Here's how the part is built. I have some questions about the finished solid (model axes, mm). A direction names the side the tool comes from. Coordinates: 2 decimals unless noted, no trailing zeros. Order: outer loops, then holes, each group sorted by start corner. A loop starts at its lowest first (then second) coordinate and runs counter-clockwise, first axis right, second up. Notation, with made-up numbers: (40.5, -21) - (60.5, -21) arc R35 cw to (60.5, 12) - close; hole circle Ø5 at (16.25, 25.5). An arc over 180 degrees is marked (long way). Answer as CSV lines item,"result". Start each with the question number.
Item 1: Imagine slicing it at A-A on y = 5. List the corners of the cut face in (x, z) for me, and give its area (3 significant figures).
Item 2: On a 3-axis mill with a long thin cutter (end or side, diameter ignored), from which of +Z, -Z, +X, -X, +Y, -Y can I reach the whole of each face in a straight line? I mean faces 1 (the face through (29.007, 27.888, 5.378)), 2 (the face through (-19.2, 27.9, 22.4)), 3 (the face through (-28, 0, 2)), 4 (the face through (25.659, 3.944, -14.557)), 5 (the face through (25.44, 3.94, 14.94)). Say none if no direction works.
Item 3: We'd pull the mould along X, two halves only. Please class faces 6 (the face through (-14, -8.5, 24)), 7 (the face through (-0.58, -12.556, 35.327)), 8 (the face through (-9.846, 27.888, -27.809)): pulls with the +X half, pulls with the -X half, needs draft (parallel to the pull), parting line crosses it, or undercut.
Item 4: Imagine slicing it at C-C on y = -7. List the corners of the cut face in (x, z) for me, and give its area (3 significant figures).
Item 5: I'm going to push flat-ended pins straight in: pin 1 (9 mm diameter, centred on x = 1.5, y = 5, fed in from -Z); pin 2 (4 mm diameter, centred on x = -25.5, z = 13.5, fed in from +Y); pin 3 (8.5 mm diameter, centred on x = 2, z = -28.5, fed in from +Y). Where does each tip first touch, or does it pass through?
Item 6: I need wall thicknesses on line 1 (Z direction, x = 0, y = 5); line 2 (X direction, y = 15, z = 0); line 3 (X direction, y = 5, z = 0). Which ranges of each line are inside material? Lowest first, please.
Item 7: Imagine slicing it at B-B on z = 30.5. List the corners of the cut face in (x, y) for me, and give its area (3 significant figures).
from build123d import *

# Parameters (mm, degrees)
EXTRUDE_1_DEPTH     = 8
SKETCH_2_R          = 27.5
EXTRUDE_2_DEPTH     = 12
EXTRUDE_3_DEPTH     = 16
SKETCH_4_R          = 29.5
EXTRUDE_4_DEPTH     = 10
FILLET_1_R          = 10
EXTRUDE_START       = 8.5
SKETCH_5_R          = 27.5
EXTRUDE_5_DEPTH     = 8.5
EXTRUDE_6_DEPTH     = 8
SKETCH_7_R          = 20
CUT_EXTRUDE_1_DEPTH = 80.671476808
FILLET_2_R          = 2
FILLET_3_R          = 2
FILLET_4_R          = 3


with BuildPart() as part:
    # Эскиз1 → Вытянуть1 (new body)
    with BuildSketch(Plane(origin=(0, 0, 0), x_dir=(1, 0, 0), z_dir=(0, 1, 0))):
        Polygon((34.063665882, 0), (17.031832941, 29.5), (-17.031832941, 29.5), (-34.063665882, 0), (-17.031832941, -29.5), (17.031832941, -29.5), align=None)
    extrude(amount=EXTRUDE_1_DEPTH)

    # Эскиз2 → Вытянуть2 (add)
    with BuildSketch(Plane(origin=(0, 8, 0), x_dir=(1, 0, 0), z_dir=(0, 1, 0))):
        with Locations(Location((0, 0, 0), (0, 0, 90))):
            Circle(SKETCH_2_R)
    extrude(amount=EXTRUDE_2_DEPTH)

    # Эскиз3 → Вытянуть3 (add)
    with BuildSketch(Plane(origin=(0, 20, 0), x_dir=(1, 0, 0), z_dir=(0, 1, 0))):
        Polygon((5.957184122, 33.538713313), (-26.066785678, 21.928429441), (-32.0239698, -11.610283872), (-5.957184122, -33.538713313), (26.066785678, -21.928429441), (32.0239698, 11.610283872), align=None)
    extrude(amount=EXTRUDE_3_DEPTH)

    # Эскиз4 → Вытянуть4 (add)
    with BuildSketch(Plane(origin=(0, 36, 0), x_dir=(1, 0, 0), z_dir=(0, 1, 0))):
        with Locations(Location((0, 0, 0), (0, 0, 109.92810259))):
            Circle(SKETCH_4_R)
    extrude(amount=EXTRUDE_4_DEPTH)

    # Скругление1
    fillet_1_edges = [part.edges().sort_by_distance(p)[0] for p in [
        (10.054800778, 46, 27.733571377),
    ]]
    fillet(fillet_1_edges, radius=FILLET_1_R - 0.0001)  # a hair under: the kernel refuses the full size

    # Эскиз5 → Вытянуть5 (add)
    with BuildSketch(Plane.XZ.offset(EXTRUDE_START)):
        with Locations(Location((0, 0, 0), (0, 0, 270))):
            Circle(SKETCH_5_R)
    extrude(amount=-EXTRUDE_5_DEPTH)

    # Эскиз6 → Вытянуть6 (add)
    with BuildSketch(Plane.XZ.offset(8.5)):
        Polygon((30.690350843, 18.423780786), (-0.610286773, 35.790513874), (-31.300637616, 17.366733088), (-30.690350843, -18.423780786), (0.610286773, -35.790513874), (31.300637616, -17.366733088), align=None)
    extrude(amount=EXTRUDE_6_DEPTH)

    # Эскиз7 → Вырез-Вытянуть1 (cut, through all)
    with BuildSketch(Plane(origin=(0, 46, 0), x_dir=(1, 0, 0), z_dir=(0, 1, 0))):
        with Locations(Location((0, 0, 0), (0, 0, 270))):
            Circle(SKETCH_7_R)
    extrude(amount=-CUT_EXTRUDE_1_DEPTH, mode=Mode.SUBTRACT)

    # Скругление2
    fillet_2_edges = [part.edges().sort_by_distance(p)[0] for p in [
        (32.0239698, 28, -11.610283872),
        (5.957184122, 28, -33.538713313),
        (-26.066785678, 28, -21.928429441),
        (-32.0239698, 28, 11.610283872),
        (-5.957184122, 28, 33.538713313),
        (26.066785678, 28, 21.928429441),
    ]]
    fillet(fillet_2_edges, radius=FILLET_2_R)

    # Скругление3
    fillet_3_edges = [part.edges().sort_by_distance(p)[0] for p in [
        (17.031832941, 4, 29.5),
        (-17.031832941, 4, 29.5),
        (-34.063665882, 4, 0),
        (-17.031832941, 4, -29.5),
        (17.031832941, 4, -29.5),
        (34.063665882, 4, 0),
    ]]
    fillet(fillet_3_edges, radius=FILLET_3_R)

    # Скругление4
    fillet_4_edges = [part.edges().sort_by_distance(p)[0] for p in [
        (31.300637616, -12.5, -17.366733088),
        (30.690350843, -12.5, 18.423780786),
        (-0.610286773, -12.5, 35.790513874),
        (-31.300637616, -12.5, 17.366733088),
        (-30.690350843, -12.5, -18.423780786),
        (0.610286773, -12.5, -35.790513874),
    ]]
    fillet(fillet_4_edges, radius=FILLET_4_R)


solid = part.part
Responses:
1,outline,"(-33.49, -1) - (-17.61, -28.5) arc R2 ccw to (-15.88, -29.5) - (15.88, -29.5) arc R2 ccw to (17.61, -28.5) - (33.49, -1) arc R2 ccw to (33.49, 1) - (17.61, 28.5) arc R2 ccw to (15.88, 29.5) - (-15.88, 29.5) arc R2 ccw to (-17.61, 28.5) - (-33.49, 1) arc R2 ccw to start; hole circle Ø40 at (0, 0)"
1,area,"1,760 mm^2"
2,face 1,"+Z, +X, +Y"
2,face 2,"+Z, -X, +Y"
2,face 3,"none"
2,face 4,"-Z, +X"
2,face 5,"+Z, +X"
3,face 6,"needs draft"
3,face 7,"parting line crosses it"
3,face 8,"pulls with the -X half"
4,outline,"circle Ø55 at (0, 0); hole circle Ø40 at (0, 0)"
4,area,"1,120 mm^2"
5,pin 1,"stops at z = -29.5"
5,pin 2,"stops at y = 42.78"
5,pin 3,"stops at y = 44.76"
6,line 1,"z = -29.5 to -20, 20 to 29.5"
6,line 2,"x = -27.5 to -20, 20 to 27.5"
6,line 3,"x = -33.75 to -20, 20 to 33.75"
7,outline,"(-9.57, 20) - (2.42, 20) - (2.42, 36) - (-9.57, 36) - close; (-9.42, -16.5) - (8.92, -16.5) - (8.92, -8.5) - (-9.42, -8.5) - close"
7,area,"339 mm^2"
